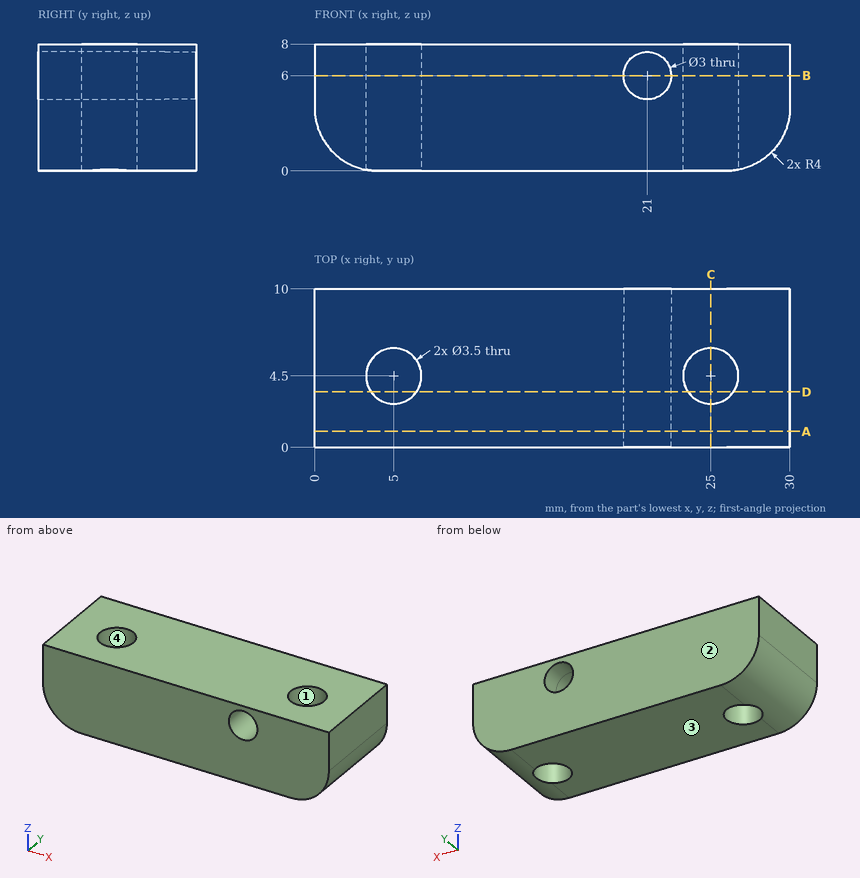
Job drawing, mm, ordinate dimensions from the low corner. One solid piece. Coordinates: 2 decimals unless noted, no trailing zeros. Write each loop counter-clockwise with the first axis right and the second up, starting at its lowest first coordinate (ties: lowest second). Pieces come first, ordered by that corner, then holes.
Item 1: Mould opens along Y. For the marked faces 1, 2, 3 and 4 say: released by +Y, released by -Y, zero draft, split by the parting line, or undercut.
Item 2: Slice it at C-C (x = 25). Write the cut outline in (y, z).
Item 3: Slice it at A-A (y = 1). Write the cut outline in (x, z).
Item 4: Slice it at B-B (z = 6). Write the cut outline in (x, y).
Item 5: Pin check, flat tips, straight feed: pin 1 (3 mm diameter, centred on x = 5, y = 4.5, fed in from -Z); pin 2 (4 mm diameter, centred on x = 21, z = 6, fed in from -Y); pin 3 (1.5 mm diameter, centred on y = 6, z = 2, fed in from +X). Stop position of each tip, or through.
Item 6: Probe line 1 (X direction, y = 9.6, z = 6); line 2 (X direction, y = 4, z = 3.5); line 3 (Y direction, x = 5, z = 4). List the from-to ranges inside material, lowest first.
Item 7: Slice it at D-D (y = 3.5). Write the cut outline in (x, z), and give its area (3 significant figures).
Results found:
1. face 1: undercut
1. face 2: released by +Y
1. face 3: zero draft
1. face 4: undercut
2. outline: (0, 0) - (2.75, 0) - (2.75, 8) - (0, 8) - close; (6.25, 0) - (10, 0) - (10, 8) - (6.25, 8) - close
3. outline: (0, 4) arc R4 ccw to (4, 0) - (26, 0) arc R4 ccw to (30, 4) - (30, 8) - (0, 8) - close; hole circle Ø3 at (21, 6)
4. outline: (0, 0) - (19.5, 0) - (19.5, 10) - (0, 10) - close; (22.5, 0) - (30, 0) - (30, 10) - (22.5, 10) - close; hole circle Ø3.5 at (5, 4.5); hole circle Ø3.5 at (25, 4.5)
5. pin 1: passes through
5. pin 2: stops at y = 0
5. pin 3: stops at x = 29.8
6. line 1: x = 0 to 19.5, 22.5 to 30
6. line 2: x = 0.03 to 3.32, 6.68 to 23.32, 26.68 to 29.97
6. line 3: y = 0 to 2.75, 6.25 to 10
7. outline: (0, 4) arc R4 ccw to (3.56, 0.02) - (3.56, 8) - (0, 8) - close; (6.44, 0) - (23.56, 0) - (23.56, 8) - (6.44, 8) - close; (26.44, 0.02) arc R4 ccw to (30, 4) - (30, 8) - (26.44, 8) - close; hole circle Ø3 at (21, 6)
7. area: 180 mm2
